Geometry check sheet. Reference: drawing and pictorial views, mm from the part's lowest x, y, z. A direction names the side the tool comes from. Round coordinates to 2 decimals unless told otherwise and drop trailing zeros. Order: outer loops, then holes, each group sorted by start corner. A loop starts at its lowest first (then second) coordinate and runs counter-clockwise, first axis right, second up.
(1) Sectioned sample at C-C (z = 4.5). Record the boundary of the cut face in (x, y), plus the area to 3 significant figures.
(2) Sectioned sample at A-A (z = 20.25). Record the boundary of the cut face in (x, y), plus the area to 3 significant figures.
(3) Material ranges on line 1 along Y through (x, z) = (74, 12.25); line 2 along Y through (x, z) = (25, 23); line 3 along X through (y, z) = (9.75, 10) (1 decimal), recorded low to high.
(4) Sectioned sample at B-B (x = 27.5). Record the boundary of the cut face in (y, z), plus the area to 3 significant figures.
(5) Set-up check for the marked faces 1, 2 and 3: record each of +Z, -Z, +X, -X, +Y, -Y from which the full face is reachable in a straight line by a thin tool's end or side.
(6) Sectioned sample at D-D (y = 14.5). Record the boundary of the cut face in (x, z) (1 decimal), plus the area to 3 significant figures.
(7) Go/stop test with flat-tipped pins: pin 1 (10 mm diameter, centred on y = 18, z = 4.5, fed in from -X) (1 decimal); pin 2 (1.5 mm diameter, centred on y = 14.5, z = 6, fed in from +X); pin 3 (5 mm diameter, centred on y = 13.5, z = 18.5, fed in from +X). Record where each tip stops, or that it passes through.
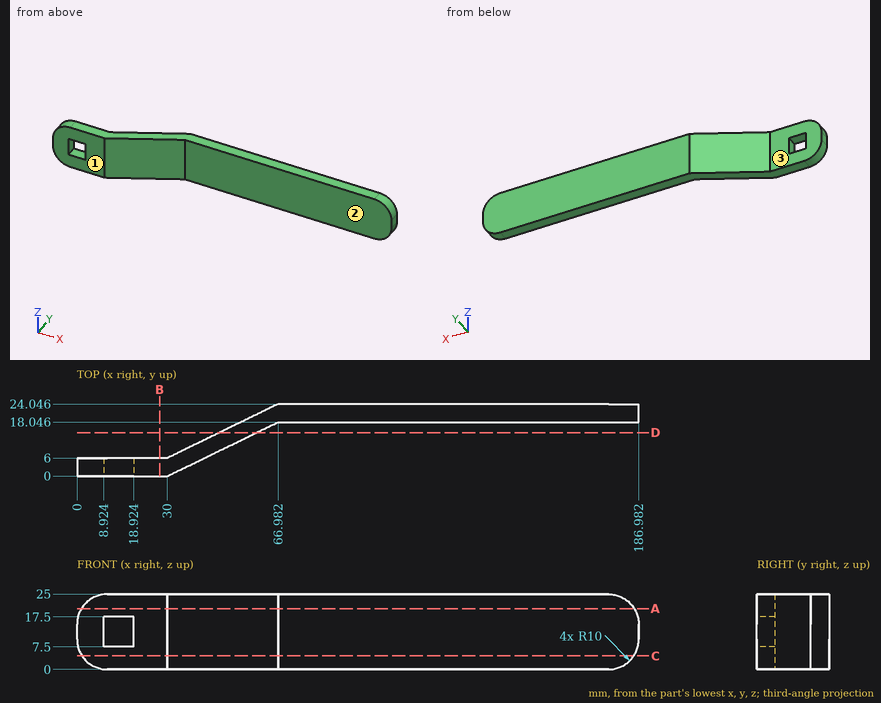
Answer below:
1. outline: (1.65, 0) - (30, 0) - (66.98, 18.05) - (185.33, 18.05) - (185.33, 24.05) - (66.98, 24.05) - (30, 6) - (1.65, 6) - close
1. area: 1,100 mm2
2. outline: (1.49, 0) - (30, 0) - (66.98, 18.05) - (185.49, 18.05) - (185.49, 24.05) - (66.98, 24.05) - (30, 6) - (1.49, 6) - close
2. area: 1,100 mm2
3. line 1: y = 18.05 to 24.05
3. line 2: y = 0 to 6
3. line 3: x = 37.7 to 50
4. outline: (0, 0) - (6, 0) - (6, 25) - (0, 25) - close
4. area: 150 mm2
5. face 1: +Z, -Z, +X, -X, -Y
5. face 2: +Z, -Z, +X, -Y
5. face 3: +Z, -Z, -X, +Y
6. outline: (47.4, 0) - (59.7, 0) - (59.7, 25) - (47.4, 25) - close
6. area: 307 mm2
7. pin 1: stops at x = 44.3
7. pin 2: stops at x = 61.25
7. pin 3: stops at x = 62.79
